from build123d import *

# Parameters (mm, degrees)
F0_W     = 7.6200012118
F0_H     = 7.6199993491
F1_DEPTH = 3.81
F2_R     = 2.2630247345
F3_DEPTH = 28.702
F4_R     = 3.4661876641
F5_DEPTH = 6.096


with BuildPart() as f1:
    # F0 (on Top) → F1 (new body, symmetric)
    with BuildSketch(Plane.XY):
        with Locations((-23.7671425566, 19.9571419507)):
            Rectangle(F0_W, F0_H)
        with Locations((23.7671425566, 19.9571419507)):
            Rectangle(F0_W, F0_H)
        with BuildLine():
            ThreePointArc((-6.8066905284, -1.2232744461), (-6.6986512028, 1.719159208), (-5.3763601299, 4.3499641462))
            Line((-5.3763601299, 4.3499641462), (-19.9571419507, 16.1471422762))
            Line((-19.9571419507, 16.1471422762), (-27.5771431625, 16.1471422762))
            Line((-27.5771431625, 16.1471422762), (-6.8066905284, -1.2232744461))
        make_face()
        with BuildLine():
            ThreePointArc((5.3763601299, 4.3499641462), (6.5195450768, 2.3071558921), (6.9157383062, 0))
            ThreePointArc((6.9157383062, 0), (6.8884224154, -0.6140626573), (6.8066905284, -1.2232744461))
            Line((6.8066905284, -1.2232744461), (27.5771431625, 16.1471422762))
            Line((27.5771431625, 16.1471422762), (19.9571419507, 16.1471422762))
            Line((19.9571419507, 16.1471422762), (5.3763601299, 4.3499641462))
        make_face()
        with BuildLine():
            Line((0, 0), (5.3763601299, 4.3499641462))
            ThreePointArc((5.3763601299, 4.3499641462), (0, 6.9157383062), (-5.3763601299, 4.3499641462))
            Line((-5.3763601299, 4.3499641462), (0, 0))
        make_face()
        with BuildLine():
            ThreePointArc((0, -6.9157383062), (4.4366423325, -5.3050580706), (6.8066905284, -1.2232744461))
            Line((6.8066905284, -1.2232744461), (0, -6.9157383062))
        make_face()
        with BuildLine():
            ThreePointArc((-6.8066905284, -1.2232744461), (-4.4366423325, -5.3050580706), (0, -6.9157383062))
            Line((0, -6.9157383062), (-6.8066905284, -1.2232744461))
        make_face()
        with BuildLine():
            ThreePointArc((6.8066905284, -1.2232744461), (6.8884224154, -0.6140626573), (6.9157383062, 0))
            ThreePointArc((6.9157383062, 0), (6.5195450768, 2.3071558921), (5.3763601299, 4.3499641462))
            Line((5.3763601299, 4.3499641462), (0, 0))
            Line((0, 0), (-5.3763601299, 4.3499641462))
            ThreePointArc((-5.3763601299, 4.3499641462), (-6.6986512028, 1.719159208), (-6.8066905284, -1.2232744461))
            Line((-6.8066905284, -1.2232744461), (0, -6.9157383062))
            Line((0, -6.9157383062), (6.8066905284, -1.2232744461))
        make_face()
    extrude(amount=F1_DEPTH, both=True)

    # F2 (on Right) → F3 (cut, symmetric)
    with BuildSketch(Plane.YZ):
        with Locations((19.9902858585, 0)):
            Circle(F2_R)
    extrude(amount=F3_DEPTH, both=True, mode=Mode.SUBTRACT)

    # F4 (on Top) → F5 (cut, symmetric)
    with BuildSketch(Plane.XY):
        Circle(F4_R)
    extrude(amount=F5_DEPTH, both=True, mode=Mode.SUBTRACT)


solid = f1.part
Design review of the part built by this model. Coordinates are the model's own, in mm. A direction names the side the tool comes from. Coordinates: 2 decimals unless noted, no trailing zeros. Write each loop counter-clockwise with the first axis right and the second up, starting at its lowest first coordinate (ties: lowest second). Pieces come first, ordered by that corner, then holes. Notation, with made-up numbers: (75, -0.5) - (86, -0.5) arc R15 ccw to (86, 23.5) - close; hole circle Ø11 at (86, 2.5). An arc over 180 degrees is marked (long way). Use one line per item in the form item = value.
Q1. Consider section A-A (x = 0). Write out the cut boundary in (y, z).
Taken from the geometry:
outline = (-6.92, -3.81) - (-3.47, -3.81) - (-3.47, 3.81) - (-6.92, 3.81) - close; (3.47, -3.81) - (6.92, -3.81) - (6.92, 3.81) - (3.47, 3.81) - close
Q2. For probe 1 along X at (y, z) = (1, 0.25); probe 2 along X at (y, z) = (10, 0.25); probe 3 along Y at (x, z) = (1, -0.5), list the stretches that pass through material, from the lowest coordinate up.
Taken from the geometry:
probe_1 = -9.47 to -3.32, 3.32 to 9.47
probe_2 = -20.23 to -12.36, 12.36 to 20.23
probe_3 = -6.84 to -3.32, 3.32 to 6.84
Q3. The part is to be moulded in two halves that separate along X. For faces 3 (the flat face through (27.577, 22, 2)), 4 (the cylindrical face through (-23.71, 17.73, 0.1)), 5 (the flat face through (19.957, 22, 2)), say which applies: +X half, -X half, draft (parallel to the pull), parting line (faces both ways), or undercut.
Taken from the geometry:
face_3 = +X half
face_4 = draft
face_5 = undercut
Q4. Insertion check: pin 1 Ø4 at (y, z) = (19.99, 0) entering from -X; pin 2 Ø2 at (x, z) = (4.5, -2) entering from +Y; pin 3 Ø8 at (x, y) = (0, 0) entering from +Z; pin 4 Ø1 at (x, z) = (13.5, 0) entering from -Y. Each pin has a flat end and moves straight along its axis. Give the tip position at first contact, or say it passes through.
Taken from the geometry:
pin_1 = through
pin_2 = 5.96
pin_3 = 3.81
pin_4 = 3.96
Q5. Machinability: for faces 1 (the flat face through (0, 6, -3.81)), 2 (the flat face through (-12.565, 10.166, 0.053)), which of the approach directions +Z, -Z, +X, -X, +Y, -Y give a long, thin tool a straight path to every point of the face, cutting with its end or side? Answer none if there is none.
Taken from the geometry:
face_1 = -Z, +X, -X, +Y, -Y
face_2 = +Z, -Z, +Y
Q6. Consider section B-B (z = 1). Write out the cut boundary in (x, y), plus the area to 3 significant figures.
Taken from the geometry:
outline = (-27.58, 16.15) - (-6.81, -1.22) arc R6.92 ccw to (6.81, -1.22) - (27.58, 16.15) - (27.58, 17.96) - (19.96, 17.96) - (19.96, 16.15) - (5.38, 4.35) arc R6.92 ccw to (-5.38, 4.35) - (-19.96, 16.15) - (-19.96, 17.96) - (-27.58, 17.96) - close; (-27.58, 22.02) - (-19.96, 22.02) - (-19.96, 23.77) - (-27.58, 23.77) - close; (19.96, 22.02) - (27.58, 22.02) - (27.58, 23.77) - (19.96, 23.77) - close; hole circle Ø6.93 at (0, 0)
area = 392 mm^2
Q7. Consider section D-D (y = 20.5). Write out the cut boundary in (x, z), plus the area to 3 significant figures.
Taken from the geometry:
outline = (-27.58, -3.81) - (-19.96, -3.81) - (-19.96, -2.2) - (-27.58, -2.2) - close; (-27.58, 2.2) - (-19.96, 2.2) - (-19.96, 3.81) - (-27.58, 3.81) - close; (19.96, -3.81) - (27.58, -3.81) - (27.58, -2.2) - (19.96, -2.2) - close; (19.96, 2.2) - (27.58, 2.2) - (27.58, 3.81) - (19.96, 3.81) - close
area = 48.9 mm^2
Q8. Consider section C-C (y = 12.5). Write out the cut boundary in (x, z).
Taken from the geometry:
outline = (-23.22, -3.81) - (-15.45, -3.81) - (-15.45, 3.81) - (-23.22, 3.81) - close; (15.45, -3.81) - (23.22, -3.81) - (23.22, 3.81) - (15.45, 3.81) - close
